Verification items for this drawing (mm, ordinates from the low corner). Give positions to 0.01 mm unless a question says otherwise; leave off trailing zeros. Loops run counter-clockwise (first coordinate to the right, second up) from the corner with the lowest first, then second, coordinate; pieces in that order, holes last. Notation, with made-up numbers: (71, -26) - (102, -26) arc R28 ccw to (102, -6) - close; hole circle Ø2 at (66.25, 42.25). An arc over 180 degrees is marked (long way). One line per question, with ' | ' between items. Start each with the question number.
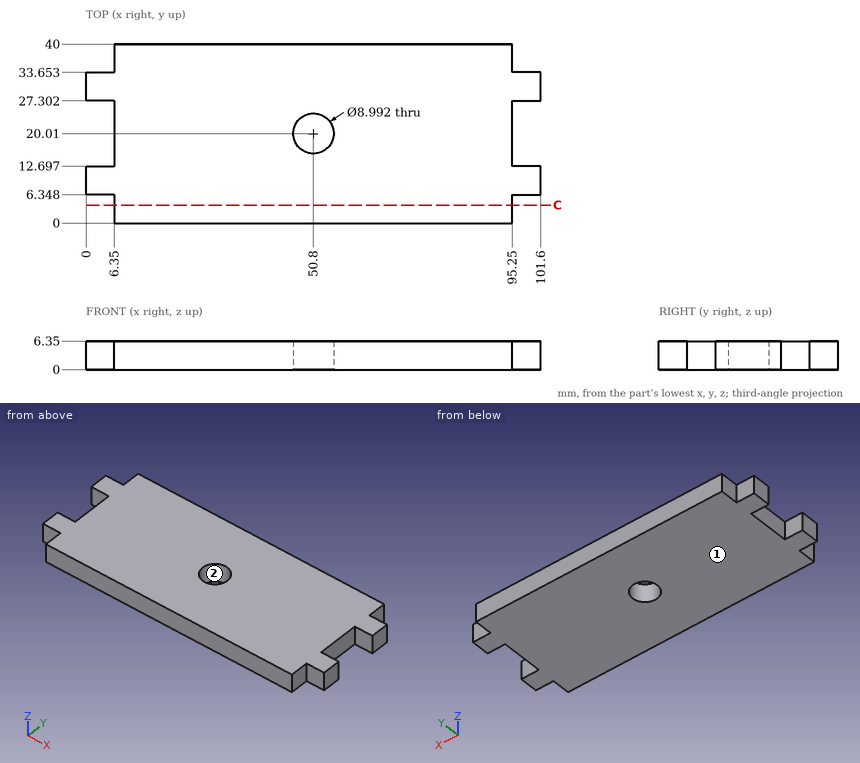
(1) Material ranges on line 1 (Y direction, x = 50.8, z = 5) (1 decimal); line 2 (X direction, y = 21.5, z = 5); line 3 (X direction, y = 17, z = 3.25), recorded low to high.
(2) Section check C-C, the plane y = 4. Record the boundary of the cut face in (x, z).
(3) Depth check by flat-ended pin: pin 1 Ø3 at (x, z) = (3.5, 4) entering from -Y; pin 2 Ø1.9 at (x, z) = (98, 2.5) entering from +Y; pin 3 Ø3 at (y, z) = (19.5, 2.5) entering from +X; pin 4 Ø2 at (x, z) = (36, 4.5) entering from -Y. Enter the tip coordinate at first touch or a pass-through.
(4) Mould release check, pull along Y, two halves, no side actions. Record for the marked faces 1 and 2: pulls with the +Y half, pulls with the -Y half, needs draft (parallel to the pull), parting line crosses it, or undercut.
Numbers:
1) line 1: 0 to 15.5, 24.5 to 40 | line 2: 6.35 to 46.56, 55.04 to 95.25 | line 3: 6.35 to 47.46, 54.14 to 95.25
2) outline: (6.35, 0) - (95.25, 0) - (95.25, 6.35) - (6.35, 6.35) - close
3) pin 1: y = 6.35 | pin 2: y = 33.65 | pin 3: x = 95.25 | pin 4: y = 0
4) face 1: needs draft | face 2: undercut
